Build history of the part. All positions in model axes, mm. Coordinates: 2 decimals unless noted, no trailing zeros. Order: outer loops, then holes, each group sorted by start corner. A loop starts at its lowest first (then second) coordinate and runs counter-clockwise, first axis right, second up. Notation, with made-up numbers: (-19, 39) - (9, 39) arc R28 ccw to (9, 70) - close; hole circle Ø7 at (83.5, -24). An arc over 180 degrees is marked (long way). One line per item, written item: value.
from build123d import *

# Parameters (mm, degrees)
ESQUISSE1_R             = 2
BOSS_EXTRU_1_DEPTH      = 3
ESQUISSE2_R             = 3
ESQUISSE2_W             = 90
ESQUISSE2_H             = 28
ENL_V_MAT_EXTRU_1_DEPTH = 3
ESQUISSE3_W             = 20
ESQUISSE3_H             = 40
ENL_V_MAT_EXTRU_2_DEPTH = 10


with BuildPart() as part:
    # Esquisse1 → Boss.-Extru.1 (new body)
    with BuildSketch(Plane.XY):
        with BuildLine():
            Line((10, 0), (105, 0))
            Line((105, 0), (105, -40))
            ThreePointArc((105, -40), (135, -70), (165, -40))
            Line((165, -40), (165, 0))
            Line((165, 0), (260, 0))
            ThreePointArc((260, 0), (267.071067812, -2.928932188), (270, -10))
            Line((270, -10), (270, -139.676541182))
            ThreePointArc((270, -139.676541182), (266.976328917, -146.976328917), (259.676541182, -150))
            Line((259.676541182, -150), (10.323458818, -150))
            ThreePointArc((10.323458818, -150), (3.023671083, -146.976328917), (0, -139.676541182))
            Line((0, -139.676541182), (0, -10))
            ThreePointArc((0, -10), (2.928932188, -2.928932188), (10, 0))
        make_face()
        with Locations((221.512678431, -88)):
            Circle(ESQUISSE1_R, mode=Mode.SUBTRACT)
        with Locations((202.512678431, -88)):
            Circle(ESQUISSE1_R, mode=Mode.SUBTRACT)
        with Locations((240.512678431, -88)):
            Circle(ESQUISSE1_R, mode=Mode.SUBTRACT)
        with Locations((221.512678431, -120)):
            Circle(ESQUISSE1_R, mode=Mode.SUBTRACT)
        with Locations((240.512678431, -120)):
            Circle(ESQUISSE1_R, mode=Mode.SUBTRACT)
        with Locations((202.512678431, -120)):
            Circle(ESQUISSE1_R, mode=Mode.SUBTRACT)
        with Locations((67.487321569, -88)):
            Circle(ESQUISSE1_R, mode=Mode.SUBTRACT)
        with Locations((48.487321569, -88)):
            Circle(ESQUISSE1_R, mode=Mode.SUBTRACT)
        with Locations((29.487321569, -88)):
            Circle(ESQUISSE1_R, mode=Mode.SUBTRACT)
        with Locations((29.487321569, -120)):
            Circle(ESQUISSE1_R, mode=Mode.SUBTRACT)
        with Locations((48.487321569, -120)):
            Circle(ESQUISSE1_R, mode=Mode.SUBTRACT)
        with Locations((67.487321569, -120)):
            Circle(ESQUISSE1_R, mode=Mode.SUBTRACT)
        with Locations((191, -121.789429788)):
            Circle(ESQUISSE1_R, mode=Mode.SUBTRACT)
        with Locations((191, -86.789429788)):
            Circle(ESQUISSE1_R, mode=Mode.SUBTRACT)
        with Locations((162.4, -86.789429788)):
            Circle(ESQUISSE1_R, mode=Mode.SUBTRACT)
        with Locations((162.4, -121.789429788)):
            Circle(ESQUISSE1_R, mode=Mode.SUBTRACT)
        with Locations((109.4, -86.789429788)):
            Circle(ESQUISSE1_R, mode=Mode.SUBTRACT)
        with Locations((109.4, -121.789429788)):
            Circle(ESQUISSE1_R, mode=Mode.SUBTRACT)
        with Locations((79, -86.789429788)):
            Circle(ESQUISSE1_R, mode=Mode.SUBTRACT)
        with Locations((79, -121.789429788)):
            Circle(ESQUISSE1_R, mode=Mode.SUBTRACT)
    extrude(amount=BOSS_EXTRU_1_DEPTH)

    # Esquisse2 → Enlèv. mat.-Extru.1 (cut)
    with BuildSketch(Plane.XY.offset(3)):
        with Locations((10, -10)):
            Circle(ESQUISSE2_R)
        with Locations((260, -10)):
            Circle(ESQUISSE2_R)
        with Locations((260, -145)):
            Circle(ESQUISSE2_R)
        with Locations((10, -145)):
            Circle(ESQUISSE2_R)
        with Locations((135, -104)):
            Rectangle(ESQUISSE2_W, ESQUISSE2_H)
    extrude(amount=-ENL_V_MAT_EXTRU_1_DEPTH, mode=Mode.SUBTRACT)

    # Esquisse3 → Enlèv. mat.-Extru.2 (cut)
    with BuildSketch(Plane.XY.offset(3)):
        with Locations((255, -70)):
            Rectangle(ESQUISSE3_W, ESQUISSE3_H)
    extrude(amount=-ENL_V_MAT_EXTRU_2_DEPTH, mode=Mode.SUBTRACT)


solid = part.part
1. Band-saw the part on C-C, the plane z = 0.7. Count the separate pieces of the cut face and the enclosed holes in it, and give its area (3 significant figures).
Values found:
separate pieces: 1
enclosed holes: 26
area: 32,900 mm2
2. Band-saw the part on A-A, the plane y = -23. Give the cut face in (x, z).
Values found:
outline: (0, 0) - (105, 0) - (105, 3) - (0, 3) - close; (165, 0) - (270, 0) - (270, 3) - (165, 3) - close
3. Two-plate mould, pull along X, no slides. Class faces 1 (the face through (257, -10, 2)), 2 (the face through (2.85, -3.01, 1.48)), 3 (the face through (267.056, -146.896, 1.479)): pulls with the +X half, pulls with the -X half, needs draft (parallel to the pull), parting line crosses it, or undercut.
Values found:
face 1: undercut
face 2: pulls with the -X half
face 3: pulls with the +X half
4. Probe line 1 along Y through (x, z) = (191, 2.3); line 2 along X through (y, z) = (-82, 0.45); line 3 along Y through (x, z) = (250.5, 0.35). List the from-to ranges inside material, lowest first.
Values found:
line 1: y = -150 to -123.79, -119.79 to -88.79, -84.79 to 0
line 2: x = 0 to 245, 265 to 270
line 3: y = -150 to -90, -50 to 0
5. Band-saw the part on B-B, the plane y = -80. Give the cut face in (x, z), and give its area (3 significant figures).
Values found:
outline: (0, 0) - (245, 0) - (245, 3) - (0, 3) - close; (265, 0) - (270, 0) - (270, 3) - (265, 3) - close
area: 750 mm2
